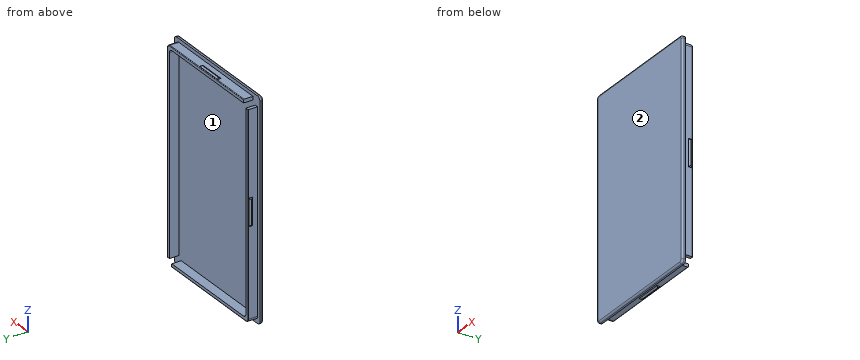
Autodesk Inventor part; units mm, degrees
ref_plane "Work Plane1" through (-67.9087, 3.175, -33.1107) normal (0, 0, 1) x (1, 0, 0)
ref_plane "Work Plane2" through (-17.2357, 3.175, 62.0123) normal (1, 0, 0) x (0, 0, -1)
ref_plane "YZ Plane" through (0, 0, 0) normal (1, 0, 0) x (0, 1, 0)
sketch "Sketch1" plane through (0, 0, 0) normal (0, 1, 0) x (-1, 0, 0)
  line L0 (-39.9143, 68.4893) -> (74.3857, 68.4893)
  line L1 (77.5607, 65.3143) -> (77.5607, -131.5357)
  line L2 (74.3857, -134.7107) -> (-39.9143, -134.7107)
  line L3 (-43.0893, -131.5357) -> (-43.0893, 65.3143)
  arc A0 (74.3857, -134.7107) -> (77.5607, -131.5357) centre (74.3857, -131.5357) ccw
  arc A1 (-43.0893, -131.5357) -> (-39.9143, -134.7107) centre (-39.9143, -131.5357) ccw
  arc A2 (-39.9143, 68.4893) -> (-43.0893, 65.3143) centre (-39.9143, 65.3143) ccw
  arc A3 (77.5607, 65.3143) -> (74.3857, 68.4893) centre (74.3857, 65.3143) ccw
  point P0 (0, 0)
  point P1 (-43.0893, 68.4893)
  point P2 (77.5607, -134.7107)
  point P3 (77.5607, 68.4893)
  point P4 (-43.0893, -134.7107)
  dimension "d0" = 203.2
  dimension "d1" = 120.65
  dimension "d16" = 3.175
extrude "Extrusion1" add sketch "Sketch1" along normal blind 3.175
sketch "Sketch2" plane through (0, 3.175, 0) normal (0, 1, 0) x (1, 0, 0)
  line L0 (-74.3857, -68.4893) -> (39.9143, -68.4893)
  line L1 (-77.5607, 131.5357) -> (-77.5607, -65.3143)
  line L2 (39.9143, 134.7107) -> (-74.3857, 134.7107)
  line L3 (43.0893, -65.3143) -> (43.0893, 131.5357)
  line L4 (-74.2587, 128.2337) -> (-74.2587, -62.0123)
  line L5 (-71.0837, -65.1873) -> (36.6123, -65.1873)
  line L6 (39.7873, -62.0123) -> (39.7873, 128.2337)
  line L7 (36.6123, 131.4087) -> (-71.0837, 131.4087)
  line L8 (-71.0837, 125.0587) -> (-71.0837, -58.8373)
  line L9 (-67.9087, -62.0123) -> (33.4373, -62.0123)
  line L10 (36.6123, -58.8373) -> (36.6123, 125.0587)
  line L11 (33.4373, 128.2337) -> (-67.9087, 128.2337)
  arc A0 (-74.2587, -62.0123) -> (-71.0837, -65.1873) centre (-71.0837, -62.0123) ccw
  arc A1 (-71.0837, -58.8373) -> (-67.9087, -62.0123) centre (-67.9087, -58.8373) ccw
  arc A2 (33.4373, -62.0123) -> (36.6123, -58.8373) centre (33.4373, -58.8373) ccw
  arc A3 (36.6123, -65.1873) -> (39.7873, -62.0123) centre (36.6123, -62.0123) ccw
  arc A4 (39.7873, 128.2337) -> (36.6123, 131.4087) centre (36.6123, 128.2337) ccw
  arc A5 (36.6123, 125.0587) -> (33.4373, 128.2337) centre (33.4373, 125.0587) ccw
  arc A6 (-67.9087, 128.2337) -> (-71.0837, 125.0587) centre (-67.9087, 125.0587) ccw
  arc A7 (-71.0837, 131.4087) -> (-74.2587, 128.2337) centre (-71.0837, 128.2337) ccw
  line L12 (-71.0837, -58.8373) -> (-74.2587, -58.8373)
  line L13 (-67.9087, -62.0123) -> (-67.9087, -65.1873)
  line L14 (36.6123, 125.0587) -> (39.7873, 125.0587)
  line L15 (33.4373, 128.2337) -> (33.4373, 131.4087)
  point P0 (0, 0)
  point P1 (-77.5607, -68.4893)
  point P2 (43.0893, -68.4893)
  point P3 (-77.5607, 134.7107)
  point P4 (43.0893, 134.7107)
  dimension "d11" = 3.302
  dimension "d12" = 3.175
  dimension "d13" = 3.175
extrude "Extrusion3" add sketch "Sketch2" along normal blind 8.89 contours A7 L7 L15 L11 A6 L8 L12 L4 | L9 A2 L10 L14 L6 A3 L5 L13
sketch "Sketch3" plane through (-74.2587, 3.175, -128.2337) normal (-1, 0, 0) x (0, 0, 1)
  line L0 (3.175, 0) -> (187.071, 0)
  line L1 (95.123, 0) -> (95.123, 6.4135)
  line L2 (82.423, 4.826) -> (107.823, 4.826)
  line L3 (107.823, 4.826) -> (107.823, 8.001)
  line L4 (107.823, 8.001) -> (82.423, 8.001)
  line L5 (82.423, 8.001) -> (82.423, 4.826)
  line L6 (82.423, 4.826) -> (107.823, 8.001) construction
  line L7 (107.823, 4.826) -> (82.423, 8.001) construction
  point P0 (128.2337, -3.175)
  dimension "d17" = 6.4135
  dimension "d18" = 25.4
  dimension "d19" = 3.175
extrude "Extrusion4" add sketch "Sketch3" along normal blind 8.255 draft -60
sketch "Sketch5" plane through (-67.9087, 3.175, 65.1873) normal (0, 0, 1) x (1, 0, 0)
  line L0 (0, 0) -> (0, 8.89)
  line L1 (101.346, 0) -> (101.346, 8.89)
  line L2 (63.373, 4.826) -> (37.973, 4.826)
  line L3 (37.973, 4.826) -> (37.973, 8.001)
  line L4 (37.973, 8.001) -> (63.373, 8.001)
  line L5 (63.373, 8.001) -> (63.373, 4.826)
  line L6 (63.373, 4.826) -> (37.973, 8.001) construction
  line L7 (37.973, 4.826) -> (63.373, 8.001) construction
  line L8 (-6.477, 0) -> (107.823, 0)
  point P0 (67.9087, -3.175)
  point P1 (50.673, 6.4135)
  dimension "d22" = 25.4
  dimension "d23" = 3.175
  dimension "d24" = 6.4135
extrude "Extrusion5" add sketch "Sketch5" along normal blind 8.89 draft -60
ref_plane "Work Plane1" through (-67.9087, 3.175, -33.1107) normal (0, 0, 1) x (1, 0, 0)
ref_plane "Work Plane2" through (-17.2357, 3.175, 62.0123) normal (1, 0, 0) x (0, 0, -1)
mirror "Mirror1" about plane through (-67.9087, 3.175, -33.1107) normal (0, 0, 1) of "Extrusion5"
mirror "Mirror2" about plane through (-17.2357, 3.175, 62.0123) normal (1, 0, 0) of "Extrusion4"
fillet "Fillet1" radius 1.5875 8 edges at (42.1594, 0, -133.7808) (-17.2357, 0, -134.7107) (-76.6308, 0, -133.7808) (-77.5607, 0, -33.1107) (-76.6308, 0, 67.5593) (-17.2357, 0, 68.4893) (42.1594, 0, 67.5593) (43.0893, 0, -33.1107)
fillet "Fillet2" radius 0.5715 6 edges at (38.8574, 12.065, 64.2573) (-15.6482, 12.065, 65.1873) (39.7873, 12.065, -31.5232) (-73.3288, 12.065, -130.4788) (-74.2587, 12.065, -34.6982) (-18.8232, 12.065, -131.4087)
properties part number "RemoteControllerBottom"
Here's how the part is built. I have some questions about the finished solid (model axes, mm). Face numbers are marked on the shaded views. Coordinates: 2 decimals unless noted, no trailing zeros. Order: outer loops, then holes, each group sorted by start corner. A loop starts at its lowest first (then second) coordinate and runs counter-clockwise, first axis right, second up. Notation, with made-up numbers: M 10.5,-6.75 L 21.5,-6.75 A33 ccw 21.5,23.25 Z; hole C -14.75,52 d9. An arc over 180 degrees is marked long. Answer as a JSON object with one key per item and string values. Group by question number.
(1) Suppose I cut it at B-B, the plane y = 5.25. Please give me the cut outline in (x, z) (3 decimals).
(2) If we mould it in two halves opening along X, with no side actions, what happens to the marked faces 1 and 2? For each: released by +X, released by -X, zero draft, split by the parting line, or undercut.
(3) Suppose I cut it at D-D, the plane z = 48. Please give me the cut outline in (x, y) (1 decimal), then the cut area to 3 significant figures.
(4) I need wall thicknesses on probe 1 along Z at (x, y) = (-26.5, 5); probe 2 along X at (y, z) = (7, 4.5); probe 3 along Y at (x, z) = (12, -122) (3 decimals). Which ranges of each line are inside material? Lowest first, please.
(5) Suppose I cut it at C-C, the plane x = 0.5. Please give me the cut outline in (y, z) (1 decimal), then the cut area to 3 significant figures.
(6) For pin 1 (3.5 mm diameter, centred on y = 8, z = 63.5, fed in from -X); pin 2 (1 mm diameter, centred on y = 6.5, z = -130.5, fed in from +X); pin 3 (1 mm diameter, centred on x = -73, y = 6, fed in from +Z), each with a flat end and sliding along its axis, tell me the tip position at first contact or that it passes through.
Values found:
{
 "1": {"outline": "M -74.259,-128.234 A3.175 ccw -71.084,-131.409 L 33.437,-131.409 L 33.437,-128.234 L -67.909,-128.234 A3.175 cw -71.084,-125.059 L -71.084,58.837 L -74.259,58.837 Z; M -67.909,62.012 L 33.437,62.012 A3.175 cw 36.612,58.837 L 36.612,-125.059 L 39.787,-125.059 L 39.787,62.012 A3.175 ccw 36.612,65.187 L -67.909,65.187 Z"},
 "2": {"face 1": "undercut", "face 2": "zero draft"},
 "3": {"outline": "M -77.6,1.6 A1.6 ccw -76,0 L 41.5,0 A1.6 ccw 43.1,1.6 L 43.1,3.2 L 39.8,3.2 L 39.8,11.5 A0.6 ccw 39.2,12.1 L 36.6,12.1 L 36.6,3.2 L -71.1,3.2 L -71.1,12.1 L -73.7,12.1 A0.6 ccw -74.3,11.5 L -74.3,3.2 L -77.6,3.2 Z", "area": "438 mm^2"},
 "4": {"probe 1": "z = -131.41 to -128.23, 62.01 to 65.19", "probe 2": "x = -74.26 to -71.08, 36.61 to 39.79", "probe 3": "y = 0 to 3.175"},
 "5": {"outline": "M 0,-133.1 A1.6 ccw 1.6,-134.7 L 3.2,-134.7 L 3.2,-131.4 L 11.5,-131.4 A0.6 ccw 12.1,-130.8 L 12.1,-128.2 L 3.2,-128.2 L 3.2,62 L 12.1,62 L 12.1,64.6 A0.6 ccw 11.5,65.2 L 3.2,65.2 L 3.2,68.5 L 1.6,68.5 A1.6 ccw 0,66.9 Z", "area": "700 mm^2"},
 "6": {"pin 1": "stops at x = -67.91", "pin 2": "stops at x = 33.44", "pin 3": "stops at z = 58.84"}
}
